```python
from build123d import *

# Parameters (mm, degrees)
BASE_FLANGE1_DEPTH      = 1.5
CUT_EXTRUDE1_DEPTH      = 11.07472084
CUT_EXTRUDE1_DEPTH_BACK = 11.07472084
SKETCH6_W               = 0.75
SKETCH6_H               = 3.25
FILLET1_R               = 0.2
FILLET2_R               = 0.25


# Sheet-metal steps are written as plain solids
with BuildPart() as part:
    # Sketch1 → Base-Flange1 (new, symmetric)
    with BuildSketch(Plane.XY):
        with BuildLine():
            Line((8.1, 0), (6.6, 0))
            ThreePointArc((6.6, 0), (6.246446609, -0.146446609), (6.1, -0.5))
            Line((6.1, -0.5), (6.1, -5.3))
            ThreePointArc((6.1, -5.3), (6.041421356, -5.441421356), (5.9, -5.5))
            Line((5.9, -5.5), (-5.9, -5.5))
            ThreePointArc((-5.9, -5.5), (-6.041421356, -5.441421356), (-6.1, -5.3))
            Line((-6.1, -5.3), (-6.1, -0.5))
            ThreePointArc((-6.1, -0.5), (-6.246446609, -0.146446609), (-6.6, 0))
            Line((-6.6, 0), (-8.1, 0))
            Line((-8.1, 0), (-8.1, -0.3))
            Line((-8.1, -0.3), (-6.6, -0.3))
            ThreePointArc((-6.6, -0.3), (-6.458578644, -0.358578644), (-6.4, -0.5))
            Line((-6.4, -0.5), (-6.4, -5.3))
            ThreePointArc((-6.4, -5.3), (-6.253553391, -5.653553391), (-5.9, -5.8))
            Line((-5.9, -5.8), (5.9, -5.8))
            ThreePointArc((5.9, -5.8), (6.253553391, -5.653553391), (6.4, -5.3))
            Line((6.4, -5.3), (6.4, -0.5))
            ThreePointArc((6.4, -0.5), (6.458578644, -0.358578644), (6.6, -0.3))
            Line((6.6, -0.3), (8.1, -0.3))
            Line((8.1, -0.3), (8.1, 0))
        make_face()
    extrude(amount=BASE_FLANGE1_DEPTH, both=True)

    # Sketch6 → Cut-Extrude1 (cut, two sides: drawn at the far end of the back side and taken through both)
    with BuildSketch(Plane(origin=(0, 0, 0), x_dir=(0, 0, -1), z_dir=(1, 0, 0)).offset(-CUT_EXTRUDE1_DEPTH_BACK)):
        with Locations((1.125, 0.875)):
            Rectangle(SKETCH6_W, SKETCH6_H)
        with Locations((-1.125, 0.875)):
            Rectangle(SKETCH6_W, SKETCH6_H)
    extrude(amount=CUT_EXTRUDE1_DEPTH + CUT_EXTRUDE1_DEPTH_BACK, mode=Mode.SUBTRACT)

    # Fillet1
    fillet1_edges = [part.edges().sort_by_distance(p)[0] for p in [
        (6.25, -0.75, -1.5),
        (-6.25, -0.75, -1.5),
        (6.25, -0.75, -0.75),
        (-6.25, -0.75, -0.75),
        (6.25, -0.75, 1.5),
        (-6.25, -0.75, 1.5),
        (6.25, -0.75, 0.75),
        (-6.25, -0.75, 0.75),
    ]]
    fillet(fillet1_edges, radius=FILLET1_R)

    # Fillet2
    fillet2_edges = [part.edges().sort_by_distance(p)[0] for p in [
        (-8.1, -0.15, -0.75),
        (8.1, -0.15, -0.75),
        (8.1, -0.15, 0.75),
        (-8.1, -0.15, 0.75),
    ]]
    fillet(fillet2_edges, radius=FILLET2_R)


solid = part.part
```
CAD build for the part. Positions are in the model's coordinates, mm. A direction names the side the tool comes from. Round coordinates to 2 decimals unless told otherwise and drop trailing zeros. Order: outer loops, then holes, each group sorted by start corner. A loop starts at its lowest first (then second) coordinate and runs counter-clockwise, first axis right, second up. Notation, with made-up numbers: (0, -38) - (49, -38) arc R17 ccw to (49, -33) - close; hole circle Ø9 at (12, 41.5). An arc over 180 degrees is marked (long way). Answer as CSV lines item,"result". Start each with the question number.
1. Drill centre lines: L1, parallel to X at y = -0.8, z = -0.7; L2, parallel to Y at x = 4.5, z = 1.4; L3, parallel to Y at x = 6.75, z = -0.3. Where is each one in solid material? Low to high. Write a range as [from, to].
2. Saw through at B-B, the plane z = -1.15. Write the cut outline in (x, y), and give its area (3 significant figures).
3. Saw through at A-A, the plane y = -1.3. Write the cut outline in (x, z).
4. Pin check, flat tips, straight feed: pin 1 (1 mm diameter, centred on x = 4.5, z = -1, fed in from +Y); pin 2 (1.2 mm diameter, centred on x = 7.5, z = 0, fed in from -Y); pin 3 (1.5 mm diameter, centred on y = -3.5, z = -0.5, fed in from -X). Stop position of each tip, or through.
5. Saw through at D-D, the plane z = -0.15. Write the cut outline in (x, y).
6. Saw through at C-C, the plane x = 5. Write the cut outline in (y, z), and give its area (3 significant figures).
7. Tool access for faces 1 (the face through (-7, -0.3, 0)), 2 (the face through (0, -5.5, 0)), 3 (the face through (6.4, -3, 0)): list every direction of +Z, -Z, +X, -X, +Y, -Y with a clear straight run to the whole face (end or side of a thin tool).
Model answer:
1,L1,"x = [-6.4, -6.1], [6.1, 6.4]"
1,L2,"y = [-5.8, -5.5]"
1,L3,"y = [-0.3, 0]"
2,outline,"(-6.4, -5.3) arc R0.5 ccw to (-5.9, -5.8) - (5.9, -5.8) arc R0.5 ccw to (6.4, -5.3) - (6.4, -0.75) - (6.1, -0.75) - (6.1, -5.3) arc R0.2 cw to (5.9, -5.5) - (-5.9, -5.5) arc R0.2 cw to (-6.1, -5.3) - (-6.1, -0.75) - (-6.4, -0.75) - close"
2,area,"6.60 mm²"
3,outline,"(-6.4, -1.5) - (-6.1, -1.5) - (-6.1, 1.5) - (-6.4, 1.5) - close; (6.1, -1.5) - (6.4, -1.5) - (6.4, 1.5) - (6.1, 1.5) - close"
4,pin 1,"stops at y = -5.5"
4,pin 2,"stops at y = -0.3"
4,pin 3,"stops at x = -6.4"
5,outline,"(-8.1, -0.3) - (-6.6, -0.3) arc R0.2 cw to (-6.4, -0.5) - (-6.4, -5.3) arc R0.5 ccw to (-5.9, -5.8) - (5.9, -5.8) arc R0.5 ccw to (6.4, -5.3) - (6.4, -0.5) arc R0.2 cw to (6.6, -0.3) - (8.1, -0.3) - (8.1, 0) - (6.6, 0) arc R0.5 ccw to (6.1, -0.5) - (6.1, -5.3) arc R0.2 cw to (5.9, -5.5) - (-5.9, -5.5) arc R0.2 cw to (-6.1, -5.3) - (-6.1, -0.5) arc R0.5 ccw to (-6.6, 0) - (-8.1, 0) - close"
6,outline,"(-5.8, -1.5) - (-5.5, -1.5) - (-5.5, 1.5) - (-5.8, 1.5) - close"
6,area,"0.900 mm²"
7,face 1,"+Z, -Z, -X, -Y"
7,face 2,"+Z, -Z, +Y"
7,face 3,"+Z, -Z, +X, -Y"
